Geometry check sheet. Reference: drawing and pictorial views, mm from the part's lowest x, y, z. Give positions to 0.01 mm unless a question says otherwise; leave off trailing zeros. Order: outer loops, then holes, each group sorted by start corner. A loop starts at its lowest first (then second) coordinate and runs counter-clockwise, first axis right, second up.
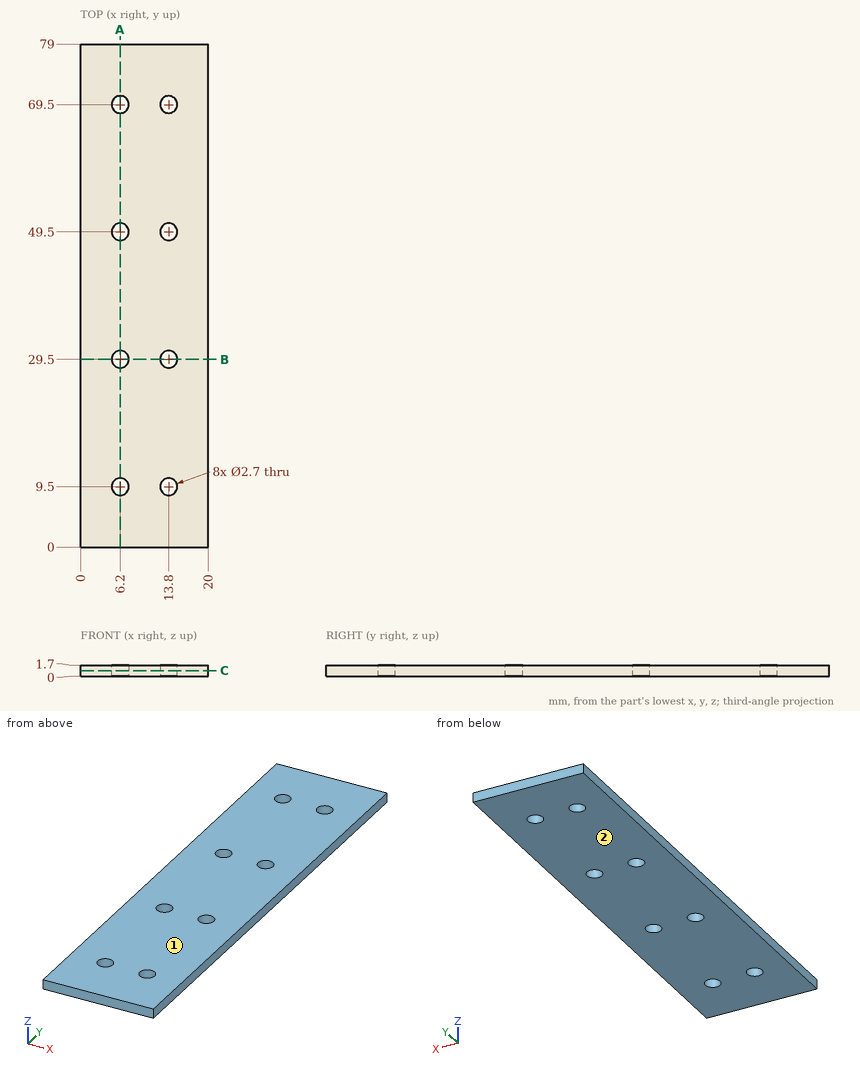
1) Depth check by flat-ended pin: pin 1 Ø3 at (x, y) = (13.8, 29.5) entering from -Z. Enter the tip coordinate at first touch or a pass-through.
Recorded:
pin 1: stops at z = 0
2) Section check A-A, the plane x = 6.2. Record the cut outline in (y, z).
Recorded:
outline: (0, 0) - (8.15, 0) - (8.15, 1.7) - (0, 1.7) - close; (10.85, 0) - (28.15, 0) - (28.15, 1.7) - (10.85, 1.7) - close; (30.85, 0) - (48.15, 0) - (48.15, 1.7) - (30.85, 1.7) - close; (50.85, 0) - (68.15, 0) - (68.15, 1.7) - (50.85, 1.7) - close; (70.85, 0) - (79, 0) - (79, 1.7) - (70.85, 1.7) - close
3) Section check C-C, the plane z = 0.85. State how many separate pieces and enclosed holes the cut face has, then the cut area to 3 significant figures.
Recorded:
separate pieces: 1
enclosed holes: 8
area: 1,530 mm2
4) Draft check along Z on the marked faces 1 and 2. Enter one of: +Z half, -Z half, draft (parallel to the pull), parting line (faces both ways), or undercut.
Recorded:
face 1: +Z half
face 2: -Z half
5) Material ranges on L1, parallel to Y at x = 6.2, z = 1; L2, parallel to X at y = 8.5, z = 0.2; L3, parallel to Y at x = 5, z = 1.6, recorded low to high.
Recorded:
L1: y = 0 to 8.15, 10.85 to 28.15, 30.85 to 48.15, 50.85 to 68.15, 70.85 to 79
L2: x = 0 to 5.29, 7.11 to 12.89, 14.71 to 20
L3: y = 0 to 8.88, 10.12 to 28.88, 30.12 to 48.88, 50.12 to 68.88, 70.12 to 79
6) Section check B-B, the plane y = 29.5. Record the cut outline in (x, z), then the cut area to 3 significant figures.
Recorded:
outline: (0, 0) - (4.85, 0) - (4.85, 1.7) - (0, 1.7) - close; (7.55, 0) - (12.45, 0) - (12.45, 1.7) - (7.55, 1.7) - close; (15.15, 0) - (20, 0) - (20, 1.7) - (15.15, 1.7) - close
area: 24.8 mm2
